CAD build for the part. Positions are in the model's coordinates, mm. Face numbers are marked on the shaded views. A direction names the side the tool comes from. Coordinates: 2 decimals unless noted, no trailing zeros. Loops run counter-clockwise (first coordinate to the right, second up) from the corner with the lowest first, then second, coordinate; pieces in that order, holes last. Notation, with made-up numbers: (25, -10) -> (32, -10) arc R30 cw to (32, 19) -> close; hole circle Ø7 at (12, 68.5). An arc over 180 degrees is marked (long way). Write each question's results on one line, items separated by ' | '.
```python
from build123d import *

# Parameters (mm, degrees)
SKETCH1_W           = 19.05
SKETCH1_H           = 38.1
SKETCH1_W_2         = 12.7
SKETCH1_H_2         = 31.75
BOSS_EXTRUDE1_DEPTH = 127
SKETCH2_R           = 1.5875
CUT_EXTRUDE1_DEPTH  = 20.05
CUT_EXTRUDE2_REACH  = 21.05
SKETCH3_R           = 4.7625
SKETCH4_R           = 1.5875
CUT_EXTRUDE3_DEPTH  = 20.05
CUT_EXTRUDE4_REACH  = 21.05
SKETCH5_R           = 4.7625


with BuildPart() as part:
    # Sketch1 → Boss-Extrude1 (new body)
    with BuildSketch(Plane(origin=(0, 0, 0), x_dir=(1, 0, 0), z_dir=(0, 1, 0))):
        with Locations((9.525, 19.05)):
            Rectangle(SKETCH1_W, SKETCH1_H)
        with Locations((9.525, 19.05)):
            Rectangle(SKETCH1_W_2, SKETCH1_H_2, mode=Mode.SUBTRACT)
    extrude(amount=BOSS_EXTRUDE1_DEPTH)

    # Sketch2 → Cut-Extrude1 (cut, through all)
    with BuildSketch(Plane(origin=(19.05, 0, 0), x_dir=(0, 0, -1), z_dir=(1, 0, 0))):
        with Locations((19.05, 12.7)):
            Circle(SKETCH2_R)
        with Locations((19.05, 32.69996)):
            Circle(SKETCH2_R)
        with Locations((19.05, 94.30004)):
            Circle(SKETCH2_R)
        with Locations((19.05, 114.3)):
            Circle(SKETCH2_R)
    extrude(amount=-CUT_EXTRUDE1_DEPTH, mode=Mode.SUBTRACT)

    # Sketch3 → Cut-Extrude2 (cut, up to next)
    with BuildSketch(Plane(origin=(19.05, 0, 0), x_dir=(0, 0, -1), z_dir=(1, 0, 0)), mode=Mode.PRIVATE) as cut_extrude2_sk1:
        with Locations((19.05, 114.3)):
            Circle(SKETCH3_R)
    cut_extrude2_tool1 = extrude(cut_extrude2_sk1.sketch, amount=-CUT_EXTRUDE2_REACH, mode=Mode.PRIVATE) & part.part
    add(cut_extrude2_tool1.solids().sort_by_distance((19.05, 114.3, -19.05))[0], mode=Mode.SUBTRACT)
    # Sketch3 → Cut-Extrude2 (cut, up to next)
    with BuildSketch(Plane(origin=(19.05, 0, 0), x_dir=(0, 0, -1), z_dir=(1, 0, 0)), mode=Mode.PRIVATE) as cut_extrude2_sk2:
        with Locations((19.05, 94.30004)):
            Circle(SKETCH3_R)
    cut_extrude2_tool2 = extrude(cut_extrude2_sk2.sketch, amount=-CUT_EXTRUDE2_REACH, mode=Mode.PRIVATE) & part.part
    add(cut_extrude2_tool2.solids().sort_by_distance((19.05, 94.30004, -19.05))[0], mode=Mode.SUBTRACT)
    # Sketch3 → Cut-Extrude2 (cut, up to next)
    with BuildSketch(Plane(origin=(19.05, 0, 0), x_dir=(0, 0, -1), z_dir=(1, 0, 0)), mode=Mode.PRIVATE) as cut_extrude2_sk3:
        with Locations((19.05, 33.059408242)):
            Circle(SKETCH3_R)
    cut_extrude2_tool3 = extrude(cut_extrude2_sk3.sketch, amount=-CUT_EXTRUDE2_REACH, mode=Mode.PRIVATE) & part.part
    add(cut_extrude2_tool3.solids().sort_by_distance((19.05, 33.059408, -19.05))[0], mode=Mode.SUBTRACT)
    # Sketch3 → Cut-Extrude2 (cut, up to next)
    with BuildSketch(Plane(origin=(19.05, 0, 0), x_dir=(0, 0, -1), z_dir=(1, 0, 0)), mode=Mode.PRIVATE) as cut_extrude2_sk4:
        with Locations((19.05, 12.7)):
            Circle(SKETCH3_R)
    cut_extrude2_tool4 = extrude(cut_extrude2_sk4.sketch, amount=-CUT_EXTRUDE2_REACH, mode=Mode.PRIVATE) & part.part
    add(cut_extrude2_tool4.solids().sort_by_distance((19.05, 12.7, -19.05))[0], mode=Mode.SUBTRACT)

    # Sketch4 → Cut-Extrude3 (cut, through all)
    with BuildSketch(Plane(origin=(19.05, 0, 0), x_dir=(0, 0, -1), z_dir=(1, 0, 0))):
        with Locations((19.05, 22.879704121)):
            Circle(SKETCH4_R)
        with Locations((19.05, 63.5)):
            Circle(SKETCH4_R)
        with Locations((19.05, 104.120295879)):
            Circle(SKETCH4_R)
    extrude(amount=-CUT_EXTRUDE3_DEPTH, mode=Mode.SUBTRACT)

    # Sketch5 → Cut-Extrude4 (cut, up to next)
    with BuildSketch(Plane.ZY, mode=Mode.PRIVATE) as cut_extrude4_sk1:
        with Locations((-19.05, 104.120295879)):
            Circle(SKETCH5_R)
    cut_extrude4_tool1 = extrude(cut_extrude4_sk1.sketch, amount=-CUT_EXTRUDE4_REACH, mode=Mode.PRIVATE) & part.part
    add(cut_extrude4_tool1.solids().sort_by_distance((0, 104.120296, -19.05))[0], mode=Mode.SUBTRACT)
    # Sketch5 → Cut-Extrude4 (cut, up to next)
    with BuildSketch(Plane.ZY, mode=Mode.PRIVATE) as cut_extrude4_sk2:
        with Locations((-19.05, 63.5)):
            Circle(SKETCH5_R)
    cut_extrude4_tool2 = extrude(cut_extrude4_sk2.sketch, amount=-CUT_EXTRUDE4_REACH, mode=Mode.PRIVATE) & part.part
    add(cut_extrude4_tool2.solids().sort_by_distance((0, 63.5, -19.05))[0], mode=Mode.SUBTRACT)
    # Sketch5 → Cut-Extrude4 (cut, up to next)
    with BuildSketch(Plane.ZY, mode=Mode.PRIVATE) as cut_extrude4_sk3:
        with Locations((-19.05, 22.879704121)):
            Circle(SKETCH5_R)
    cut_extrude4_tool3 = extrude(cut_extrude4_sk3.sketch, amount=-CUT_EXTRUDE4_REACH, mode=Mode.PRIVATE) & part.part
    add(cut_extrude4_tool3.solids().sort_by_distance((0, 22.879704, -19.05))[0], mode=Mode.SUBTRACT)


solid = part.part
```
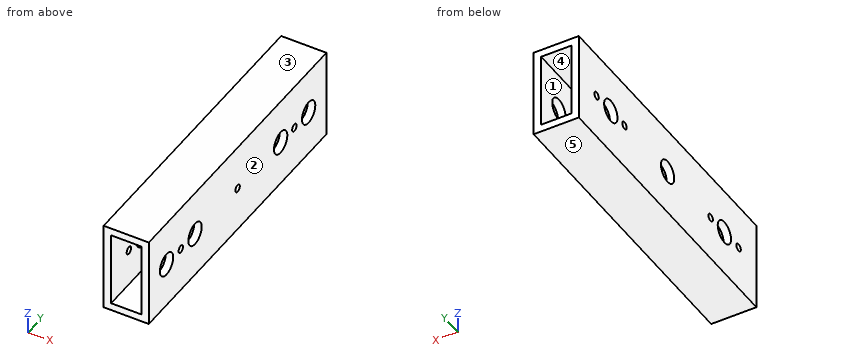
Q1. Cut at A-A on x = 10.25. Write the cut outline in (y, z) (3 decimals), and give its area (3 significant figures).
Results are:
outline: (0, -38.1) -> (127, -38.1) -> (127, -34.925) -> (0, -34.925) -> close; (0, -3.175) -> (127, -3.175) -> (127, 0) -> (0, 0) -> close | area: 806 mm^2
Q2. Which spindle directions (+Z, -Z, +X, -X, +Y, -Y) get a long thin tool onto all of the face, cutting with end or side? Do the marked faces 1 and 2. Say none if no direction does.
Results are:
face 1: +Y, -Y | face 2: +Z, -Z, +X, +Y, -Y
Q3. Wall check: L1, parallel to X at y = 31, z = -26.5 (3 decimals); L2, parallel to Y at x = 16.25, z = -15.5; L3, parallel to Z at x = 4.5, y = 22 (3 decimals). Give the ranges that are in metal, low to high. Write a range as from..to.
Results are:
L1: 0..3.175, 15.875..19.05 | L2: 0..9.53, 15.87..29.88, 36.23..91.13, 97.47..111.13, 117.47..127 | L3: -38.1..-34.925, -3.175..0
Q4. Drop flat-ended pins along their axis: pin 1 (4 mm diameter, centred on y = 63.5, z = -19.05, fed in from -X) (3 decimals); pin 2 (1.9 mm diameter, centred on y = 114.3, z = -19.05, fed in from -X). Give the stop position or say it passes through.
Results are:
pin 1: x = 15.875 | pin 2: through
Q5. Pull direction Z, two halves, no side cores. Call the marked faces 3, 4 and 5: +Z half, -Z half, draft (parallel to the pull), parting line (faces both ways), or undercut.
Results are:
face 3: +Z half | face 4: undercut | face 5: -Z half
Q6. Cut at D-D on y = 82. Write the cut outline in (x, z) (3 decimals).
Results are:
outline: (0, -38.1) -> (19.05, -38.1) -> (19.05, 0) -> (0, 0) -> close; hole (3.175, -34.925) -> (15.875, -34.925) -> (15.875, -3.175) -> (3.175, -3.175) -> close
Q7. Cut at B-B on z = -7.5. Write the cut outline in (x, y) (3 decimals).
Results are:
outline: (0, 0) -> (3.175, 0) -> (3.175, 127) -> (0, 127) -> close; (15.875, 0) -> (19.05, 0) -> (19.05, 127) -> (15.875, 127) -> close
